Work out the finished part from the listing and answer in its coordinate system (mm). A direction names the side the tool comes from. Round coordinates to 2 decimals unless told otherwise and drop trailing zeros. Write each loop counter-clockwise with the first axis right and the second up, starting at its lowest first coordinate (ties: lowest second). Pieces come first, ordered by that corner, then holes. Notation, with made-up numbers: (53.5, 51.5) -> (65.5, 51.5) arc R27 cw to (65.5, 70.5) -> close; hole circle Ø6 at (-3.5, 1.5). An arc over 180 degrees is marked (long way). Answer as a JSON object with one key per item and string values. Group by question number.
from build123d import *

# Parameters (mm, degrees)
SKETCH_1_R      = 10
EXTRUDE_2_DEPTH = 2
SKETCH_1_6_R    = 2
EXTRUDE_5_DEPTH = 50
SKETCH_8_W      = 6.431791907
SKETCH_8_H      = 4.68965636
SKETCH_8_W_2    = 4.511669879
SKETCH_8_H_2    = 3.190584844
EXTRUDE_7_DEPTH = 5
SKETCH_10_R     = 0.2
EXTRUDE_8_DEPTH = 4
SKETCH_11_R     = 2.5
EXTRUDE_9_DEPTH = 22


with BuildPart() as part:
    # Sketch 1 → Extrude 2 (new body)
    with BuildSketch(Plane(origin=(0, 0, 0), x_dir=(1, 0, 0), z_dir=(0, 1, 0))):
        with Locations(Location((5.012427746, -3.423121387, 0), (0, 0, 270))):
            Circle(SKETCH_1_R)
    extrude(amount=EXTRUDE_2_DEPTH)

    # Sketch 1_6 → Extrude 5 (add)
    with BuildSketch(Plane(origin=(0, 0, 0), x_dir=(1, 0, 0), z_dir=(0, 1, 0))):
        Polygon((-16.137572254, -21.639017341), (-16.137572254, 14.792774566), (-13.203468208, 17.726878613), (23.228323699, 17.726878613), (26.162427746, 14.792774566), (26.162427746, -21.639017341), (23.228323699, -24.573121387), (-13.203468208, -24.573121387), align=None)
        with Locations(Location((-8.722572254, -17.158121387, 0), (0, 0, 270))):
            Circle(SKETCH_1_6_R, mode=Mode.SUBTRACT)
        with Locations(Location((-8.722572254, 10.311878613, 0), (0, 0, 270))):
            Circle(SKETCH_1_6_R, mode=Mode.SUBTRACT)
        with Locations(Location((18.747427746, -17.158121387, 0), (0, 0, 270))):
            Circle(SKETCH_1_6_R, mode=Mode.SUBTRACT)
        with Locations(Location((18.747427746, 10.311878613, 0), (0, 0, 270))):
            Circle(SKETCH_1_6_R, mode=Mode.SUBTRACT)
    extrude(amount=-EXTRUDE_5_DEPTH)

    # Sketch 8 → Extrude 7 (add)
    with BuildSketch(Plane(origin=(0, 0, -17.726878613), x_dir=(-1, 0, 0), z_dir=(0, 0, -1))):
        with Locations((-5.012427746, -47.65517182)):
            Rectangle(SKETCH_8_W, SKETCH_8_H)
        with Locations((-5.085720746, -47.740684826)):
            Rectangle(SKETCH_8_W_2, SKETCH_8_H_2, mode=Mode.SUBTRACT)
    extrude(amount=EXTRUDE_7_DEPTH)

    # Sketch 10 → Extrude 8 (add)
    with BuildSketch(Plane(origin=(0, 0, -17.726878613), x_dir=(-1, 0, 0), z_dir=(0, 0, -1))):
        with Locations(Location((-6.597292785, -47.769314004, 0), (0, 0, 180))):
            Circle(SKETCH_10_R)
        with Locations(Location((-5.521254618, -47.769314004, 0), (0, 0, 180))):
            Circle(SKETCH_10_R)
        with Locations(Location((-4.574749057, -47.769314004, 0), (0, 0, 180))):
            Circle(SKETCH_10_R)
        with Locations(Location((-3.590639555, -47.769314004, 0), (0, 0, 180))):
            Circle(SKETCH_10_R)
    extrude(amount=EXTRUDE_8_DEPTH)

    # Sketch 11 → Extrude 9 (add)
    with BuildSketch(Plane(origin=(0, 2, 0), x_dir=(1, 0, 0), z_dir=(0, 1, 0))):
        with Locations(Location((5.012427746, -3.423121387, 0), (0, 0, 270))):
            Circle(SKETCH_11_R)
    extrude(amount=EXTRUDE_9_DEPTH)


solid = part.part
1) A cutting plane is placed at C-C on y = -16. Determine the outline of the cut face in (x, z).
2) Straight lines are drawn through the part: L1, parallel to Z at x = 20, y = -29.5; L2, parallel to Z at x = -9, y = -39.5; L3, parallel to X at y = -12, z = 19. For each, find the intervals that lie inside material, in ascending order.
3) A tool of negligible diameter and unlimited length cuts with its end or side. For faces 5 (the face through (5, -45.31, -20)), 6 (the face through (3, 2, 6)), 7 (the face through (1.797, -48, -20)), 8 (the face through (-8.63, -24.65, -12.31)), 9 (the face through (7.342, -48, -20)), from which of +Z, -Z, +X, -X, +Y, -Y can it reach the whole face along a straight path? Write none if from no direction.
4) A cutting plane is placed at B-B on z = -5. Determine the outline of the cut face in (x, y), plus the area to 3 significant figures.
5) A cutting plane is placed at D-D on x = -2. Determine the outline of the cut face in (y, z), plus the area to 3 significant figures.
6) A cutting plane is placed at A-A on z = -19. Determine the outline of the cut face in (x, y).
7) For a pull along Z with two mould halves and no side action, classify faces 1 (the face through (-14.65, -24.65, 23.127)), 2 (the face through (20.73, -24.65, 16.9)), 3 (the face through (8.228, -48, -20)), 4 (the face through (-4.75, 0.99, 1.26)) as released by +Z, released by -Z, zero draft, split by the parting line, or undercut.
8) Each of these flat-tipped pins is pushed along its axis until it touches: P1, Ø5, axis at x = 5, z = -3, coming from the +Y side; P2, Ø1, axis at x = 10, z = -7.5, coming from the +Y side; P3, Ø2.5, axis at y = -48, z = -20, coming from the +X side; P4, Ø3, axis at x = 18.75, z = -10.31, coming from the -Y side. Where does it stop, or does it pass through?
Established:
{
 "1": {"outline": "(-16.14, -14.79) -> (-13.2, -17.73) -> (23.23, -17.73) -> (26.16, -14.79) -> (26.16, 21.64) -> (23.23, 24.57) -> (-13.2, 24.57) -> (-16.14, 21.64) -> close; hole circle Ø4 at (-8.72, -10.31); hole circle Ø4 at (-8.72, 17.16); hole circle Ø4 at (18.75, -10.31); hole circle Ø4 at (18.75, 17.16)"},
 "2": {"L1": "z = -17.73 to -11.87, -8.75 to 15.6, 18.72 to 24.57", "L2": "z = -17.73 to -12.29, -8.33 to 15.18, 19.14 to 24.57", "L3": "x = -16.14 to -9.5, -7.94 to 17.97, 19.53 to 26.16"},
 "3": {"face 5": "-Z, +X, -X, +Y", "face 6": "+Y", "face 7": "-Z, -X, +Y, -Y", "face 8": "+Y, -Y", "face 9": "-Z"},
 "4": {"outline": "(-16.14, -50) -> (26.16, -50) -> (26.16, 0) -> (10.4, 0) -> (10.4, 2) -> (-0.38, 2) -> (-0.38, 0) -> (-16.14, 0) -> close", "area": "2,140 mm²"},
 "5": {"outline": "(-50, -17.73) -> (0, -17.73) -> (0, -3.71) -> (2, -3.71) -> (2, 10.55) -> (0, 10.55) -> (0, 24.57) -> (-50, 24.57) -> close", "area": "2,140 mm²"},
 "6": {"outline": "(1.8, -50) -> (8.23, -50) -> (8.23, -45.31) -> (1.8, -45.31) -> close; circle Ø0.4 at (3.59, -47.77); circle Ø0.4 at (4.57, -47.77); circle Ø0.4 at (5.52, -47.77); circle Ø0.4 at (6.6, -47.77); hole (2.83, -49.34) -> (7.34, -49.34) -> (7.34, -46.15) -> (2.83, -46.15) -> close"},
 "7": {"face 1": "released by +Z", "face 2": "undercut", "face 3": "zero draft", "face 4": "split by the parting line"},
 "8": {"P1": "stops at y = 2", "P2": "stops at y = 0", "P3": "stops at x = 8.23", "P4": "passes through"}
}
